```python
from build123d import *

# Parameters (mm, degrees)
SKETCH1_W           = 1676.4
SKETCH1_H           = 1066.8
BOSS_EXTRUDE1_DEPTH = 304.8
SKETCH2_W           = 1066.8
SKETCH2_H           = 1524
BOSS_EXTRUDE2_DEPTH = 304.8
FILLET1_R           = 533.4
SKETCH5_W           = 1371.6
SKETCH5_H           = 304.8
BOSS_EXTRUDE3_DEPTH = 1066.8
CUT_EXTRUDE1_DEPTH  = 1066.8
CHAMFER1_SIZE       = 304.8


with BuildPart() as part:
    # Sketch1 → Boss-Extrude1 (new body)
    with BuildSketch(Plane(origin=(0, 0, 0), x_dir=(1, 0, 0), z_dir=(0, 1, 0))):
        with Locations((838.2, 533.4)):
            Rectangle(SKETCH1_W, SKETCH1_H)
    extrude(amount=BOSS_EXTRUDE1_DEPTH)

    # Sketch2 → Boss-Extrude2 (add)
    with BuildSketch(Plane.ZY):
        with Locations((-533.4, 762)):
            Rectangle(SKETCH2_W, SKETCH2_H)
    extrude(amount=-BOSS_EXTRUDE2_DEPTH)

    # Fillet1
    fillet1_edges = [part.edges().sort_by_distance(p)[0] for p in [
        (152.4, 1524, -1066.8),
        (152.4, 1524, 0),
    ]]
    fillet(fillet1_edges, radius=FILLET1_R - 0.0001)  # a hair under: the kernel refuses the full size

    # Sketch5 → Boss-Extrude3 (add)
    with BuildSketch(Plane(origin=(0, 304.8, 0), x_dir=(1, 0, 0), z_dir=(0, 1, 0))):
        with Locations((990.6, 533.4)):
            Rectangle(SKETCH5_W, SKETCH5_H)
    extrude(amount=BOSS_EXTRUDE3_DEPTH)

    # Sketch6 → Cut-Extrude1 (cut)
    with BuildSketch(Plane.XY.offset(-381)):
        Polygon((304.8, 1371.6), (1676.4, 304.8), (1676.4, 1371.6), align=None)
    extrude(amount=-CUT_EXTRUDE1_DEPTH, mode=Mode.SUBTRACT)

    # Chamfer1
    chamfer1_edges = [part.edges().sort_by_distance(p)[0] for p in [
        (1676.4, 152.4, -1066.8),
        (1676.4, 152.4, 0),
    ]]
    chamfer(chamfer1_edges, length=CHAMFER1_SIZE)


solid = part.part
```
Build history of the part. All positions in model axes, mm. A direction names the side the tool comes from. Round coordinates to 2 decimals unless told otherwise and drop trailing zeros. Write each loop counter-clockwise with the first axis right and the second up, starting at its lowest first coordinate (ties: lowest second). Pieces come first, ordered by that corner, then holes. Notation, with made-up numbers: (48, 20) - (97, 20) arc R12 cw to (97, 32) - close; hole circle Ø1 at (56.5, 40.25). An arc over 180 degrees is marked (long way). Answer as CSV lines item,"result".
Q1. Drop flat-ended pins along their axis: pin 1 (5 mm diameter, centred on x = 466, z = -494.5, fed in from +Y); pin 2 (10 mm diameter, centred on y = 907, z = -807, fed in from +X); pin 3 (8 mm diameter, centred on x = 444, y = 692.5, fed in from -Z). Give the stop position or say it passes through.
Report:
pin 1,"stops at y = 1248.17"
pin 2,"stops at x = 304.8"
pin 3,"stops at z = -685.8"
Q2. Tool access for faces 1 (the flat face through (829, 712, -381)), 2 (the flat face through (829, 712, -685.8)), 3 (the flat face through (304.8, 923, -304)): list every direction of +Z, -Z, +X, -X, +Y, -Y with a clear straight run to the whole face (end or side of a thin tool).
Report:
face 1,"+Z, +X, +Y"
face 2,"-Z, +X, +Y"
face 3,"+X, +Y"
Q3. Cut at C-C (z = -181). Write the cut outline in (x, y), and give its area (3 significant figures).
Report:
outline,"(0, 0) - (1552.6, 0) - (1552.6, 304.8) - (304.8, 304.8) - (304.8, 1391.01) - (0, 1391.01) - close"
area,"804,000 mm^2"
Q4. Drill centre lines: probe 1 along Y at (x, z) = (1297, -157); probe 2 along Z at (x, y) = (483.5, 615). Where is each one in solid material? Low to high. Write a range as [from, to].
Report:
probe 1,"y = [0, 304.8]"
probe 2,"z = [-685.8, -381]"
Q5. Cut at D-D (z = -559). Write the cut outline in (x, y), and give its area (3 significant figures).
Report:
outline,"(0, 0) - (1676.4, 0) - (1676.4, 304.8) - (304.8, 1371.6) - (304.8, 1523.39) - (0, 1523.39) - close"
area,"1,610,000 mm^2"
Q6. Cut at A-A (y = 771). Write the cut outline in (x, z).
Report:
outline,"(0, -1066.8) - (304.8, -1066.8) - (304.8, -685.8) - (1077, -685.8) - (1077, -381) - (304.8, -381) - (304.8, 0) - (0, 0) - close"
Q7. Cut at B-B (x = 413). Write the cut outline in (y, z), and give its area (3 significant figures).
Report:
outline,"(0, -1066.8) - (304.8, -1066.8) - (304.8, -685.8) - (1287.44, -685.8) - (1287.44, -381) - (304.8, -381) - (304.8, 0) - (0, 0) - close"
area,"625,000 mm^2"
